Input: part model. Units: mm. Frame: model coordinates. A direction names the side the tool comes from. Coordinates: 2 decimals unless noted, no trailing zeros. Loops run counter-clockwise (first coordinate to the right, second up) from the corner with the lowest first, then second, coordinate; pieces in that order, holes last. Notation, with made-up numbers: M 27,21.5 L 73,21.5 A24 cw 73,42.5 Z; hole C -20.75,37.5 d10. An arc over 180 degrees is marked long. Use a Markdown table: item, result. Add a question column.
1. Section C-C on y = -7. Output: boundary loops of the cut face in (x, z).
2. Section A-A on x = 0. Output: boundary loops of the cut face in (y, z).
3. Set-up query: faces 1 (the cylindrical face through (6.642, -6.113, 18.014)), 2 (the cylindrical face through (-3.848, -17.328, 0.266)). Return all of +Z, -Z, +X, -X, +Y, -Y with unobstructed straight access to the full face (end or side cutting, diameter ignored); none if empty.
4. Line query: L1, parallel to Y at x = 0, z = 17.75; L2, parallel to Z at x = -14, y = 0; L3, parallel to Y at x = 0, z = 12. Output: solid intervals per line, ascending. Write a range as [from, to].
5. Section B-B on z = 26. Output: boundary loops of the cut face in (x, y).
6. Section D-D on x = 9. Output: boundary loops of the cut face in (y, z), then the cut area to 3 significant figures.
7. Pin query (flat end, axial travel): pin 1 (12 mm diameter, centred on x = 10, z = -6.5, fed in from -Y); pin 2 (8 mm diameter, centred on y = -11.5, z = -13.5, fed in from +X); pin 3 (1.5 mm diameter, centred on y = 7.5, z = 3.5, fed in from -X). Return the tip coordinate at first contact, or that it passes through.
```python
from build123d import *

# Parameters (mm, degrees)
SKETCH1_R           = 17.75
BOSS_EXTRUDE1_DEPTH = 19
SKETCH2_R           = 3
BOSS_EXTRUDE2_DEPTH = 10
SKETCH3_R           = 1
CUT_EXTRUDE1_DEPTH  = 2
CIRPATTERN1_COUNT   = 6
CIRPATTERN1_ANGLE   = 335


with BuildPart() as part:
    # Sketch1 → Boss-Extrude1 (new body, symmetric)
    with BuildSketch(Plane.XY):
        Circle(SKETCH1_R)
    extrude(amount=BOSS_EXTRUDE1_DEPTH, both=True)

    # Sketch2 → Boss-Extrude2 (add)
    with BuildSketch(Plane.XY.offset(19)):
        Circle(SKETCH2_R)
    extrude(amount=BOSS_EXTRUDE2_DEPTH)

    # Sketch3 → Cut-Extrude1 (cut)
    with BuildSketch(Plane.XY.offset(19)):
        with Locations((0, 10)):
            Circle(SKETCH3_R)
    cut_extrude1 = extrude(amount=-CUT_EXTRUDE1_DEPTH, mode=Mode.SUBTRACT)

    # CirPattern1: Cut-Extrude1 ×6 about axis
    cirpattern1_axis = Axis((0, 0, 0), (0, 0, -1))
    for i in range(1, CIRPATTERN1_COUNT):
        add(cut_extrude1.rotate(cirpattern1_axis, i * CIRPATTERN1_ANGLE / (CIRPATTERN1_COUNT - 1)), mode=Mode.SUBTRACT)


solid = part.part
```
Answers below:
| question | item | result |
|---|---|---|
| 1 | outline | M -16.31,-19 L 16.31,-19 L 16.31,19 L 8.19,19 L 8.19,17 L 6.19,17 L 6.19,19 L -16.31,19 Z |
| 2 | outline | M -17.75,-19 L 17.75,-19 L 17.75,19 L 11,19 L 11,17 L 9,17 L 9,19 L 3,19 L 3,29 L -3,29 L -3,19 L -17.75,19 Z |
| 3 | face 1 | +Z |
| 3 | face 2 | +Z, -Z |
| 4 | L1 | y = [-17.75, 9], [11, 17.75] |
| 4 | L2 | z = [-19, 19] |
| 4 | L3 | y = [-17.75, 17.75] |
| 5 | outline | C 0,0 d6 |
| 6 | outline | M -15.3,-19 L 15.3,-19 L 15.3,19 L 4.89,19 L 4.89,17 L 2.93,17 L 2.93,19 L -15.3,19 Z |
| 6 | area | 1,160 mm² |
| 7 | pin 1 | stops at y = -17.29 |
| 7 | pin 2 | stops at x = 16.09 |
| 7 | pin 3 | stops at x = -16.42 |
